The listing builds one solid part. Answer for the finished solid, in the listing's coordinates (mm). Face numbers are marked on the shaded views. A direction names the side the tool comes from. Give positions to 0.01 mm unless a question says otherwise; leave off trailing zeros. Write each loop counter-clockwise with the first axis right and the second up, starting at its lowest first coordinate (ties: lowest second). Pieces come first, ordered by that corner, then holes.
```python
from build123d import *

# Parameters (mm, degrees)
SKETCH1_R           = 1.371428571
BOSS_EXTRUDE1_DEPTH = 4
FILLET1_R           = 10


with BuildPart() as part:
    # Sketch1 → Boss-Extrude1 (new body)
    with BuildSketch(Plane(origin=(0, 0, 0), x_dir=(0, 0, -1), z_dir=(1, 0, 0))):
        with BuildLine():
            Line((18, 1.714285714), (25.030770044, 1.714285714))
            ThreePointArc((25.030770044, 1.714285714), (31.428571429, 0), (25.030770044, -1.714285714))
            Line((25.030770044, -1.714285714), (18, -1.714285714))
            Line((18, -1.714285714), (2.969229956, -1.714285714))
            ThreePointArc((2.969229956, -1.714285714), (-3.428571429, 0), (2.969229956, 1.714285714))
            Line((2.969229956, 1.714285714), (18, 1.714285714))
        make_face()
        Circle(SKETCH1_R, mode=Mode.SUBTRACT)
        with Locations((28, 0)):
            Circle(SKETCH1_R, mode=Mode.SUBTRACT)
    extrude(amount=BOSS_EXTRUDE1_DEPTH)

    # Fillet1
    fillet1_edges = [part.edges().sort_by_distance(p)[0] for p in [
        (2, 1.714285714, -25.030770044),
        (2, -1.714285714, -25.030770044),
        (2, -1.714285714, -2.969229956),
        (2, 1.714285714, -2.969229956),
    ]]
    fillet(fillet1_edges, radius=FILLET1_R)


solid = part.part
```
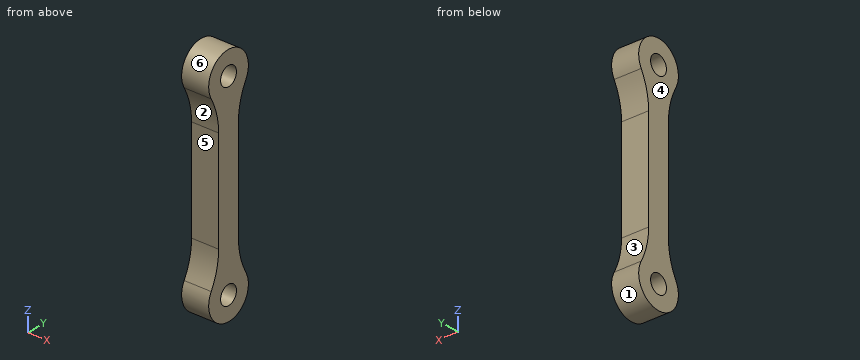
Item 1: A cutting plane is placed at D-D, the plane y = -2.5. Give the vertices of the cut face in (x, z), plus the area to 3 significant figures.
Conclusion:
outline: (0, -30.35) - (4, -30.35) - (4, -25.32) - (0, -25.32) - close; (0, -2.68) - (4, -2.68) - (4, 2.35) - (0, 2.35) - close
area: 40.2 mm2
Item 2: Consider probe 1 along Y at (x, z) = (1.6, 0); probe 2 along Z at (x, y) = (2.05, 1.25); probe 3 along Y at (x, z) = (2.9, -20). Determine where each line is inside the solid, lowest interval first.
Conclusion:
probe 1: y = -3.43 to -1.37, 1.37 to 3.43
probe 2: z = -31.19 to -28.56, -27.44 to -0.56, 0.56 to 3.19
probe 3: y = -1.71 to 1.71
Item 3: A cutting plane is placed at B-B, the plane y = 0. Give the vertices of the cut face in (x, z), plus the area to 3 significant figures.
Conclusion:
outline: (0, -31.43) - (4, -31.43) - (4, -29.37) - (0, -29.37) - close; (0, -26.63) - (4, -26.63) - (4, -1.37) - (0, -1.37) - close; (0, 1.37) - (4, 1.37) - (4, 3.43) - (0, 3.43) - close
area: 117 mm2
Item 4: Each of these flat-tipped pins is pushed along its axis until it touches: P1, Ø1.2, axis at x = 2.5, z = -14, coming from the +Y side; P2, Ø2, axis at x = 1.5, y = 1.5, coming from the -Z side; P3, Ø2, axis at x = 2.5, z = -13, coming from the -Y side. Where does it stop, or does it pass through?
Conclusion:
P1: stops at y = 1.71
P2: stops at z = -31.39
P3: stops at y = -1.71
Item 5: Which of the six approach directions +Z, -Z, +X, -X, +Y, -Y give full straight-line access (tool end or side, diameter ignored) to the marked faces 1, 2 and 3?
Conclusion:
face 1: +X, -X
face 2: +X, -X, -Y
face 3: +X, -X, +Y
Item 6: A cutting plane is placed at C-C, the plane x = 2.75. Give the vertices of the cut face in (y, z), plus the area to 3 significant figures.
Conclusion:
outline: (-2.99, -26.32) arc R3.43 ccw (long way) to (2.99, -26.32) arc R10 cw to (1.71, -21.43) - (1.71, -6.57) arc R10 cw to (2.99, -1.68) arc R3.43 ccw (long way) to (-2.99, -1.68) arc R10 cw to (-1.71, -6.57) - (-1.71, -21.43) arc R10 cw to start; hole circle Ø2.74 at (0, -28); hole circle Ø2.74 at (0, 0)
area: 140 mm2
Item 7: Determine the mould class of the marked faces 4, 5 and 6 for opening direction Z: pulls with the +Z half, pulls with the -Z half, needs draft (parallel to the pull), parting line crosses it, or undercut.
Conclusion:
face 4: needs draft
face 5: undercut
face 6: undercut
Item 8: A cutting plane is placed at A-A, the plane z = -28. Give the vertices of the cut face in (x, y), plus the area to 3 significant figures.
Conclusion:
outline: (0, -3.43) - (4, -3.43) - (4, -1.37) - (0, -1.37) - close; (0, 1.37) - (4, 1.37) - (4, 3.43) - (0, 3.43) - close
area: 16.5 mm2
